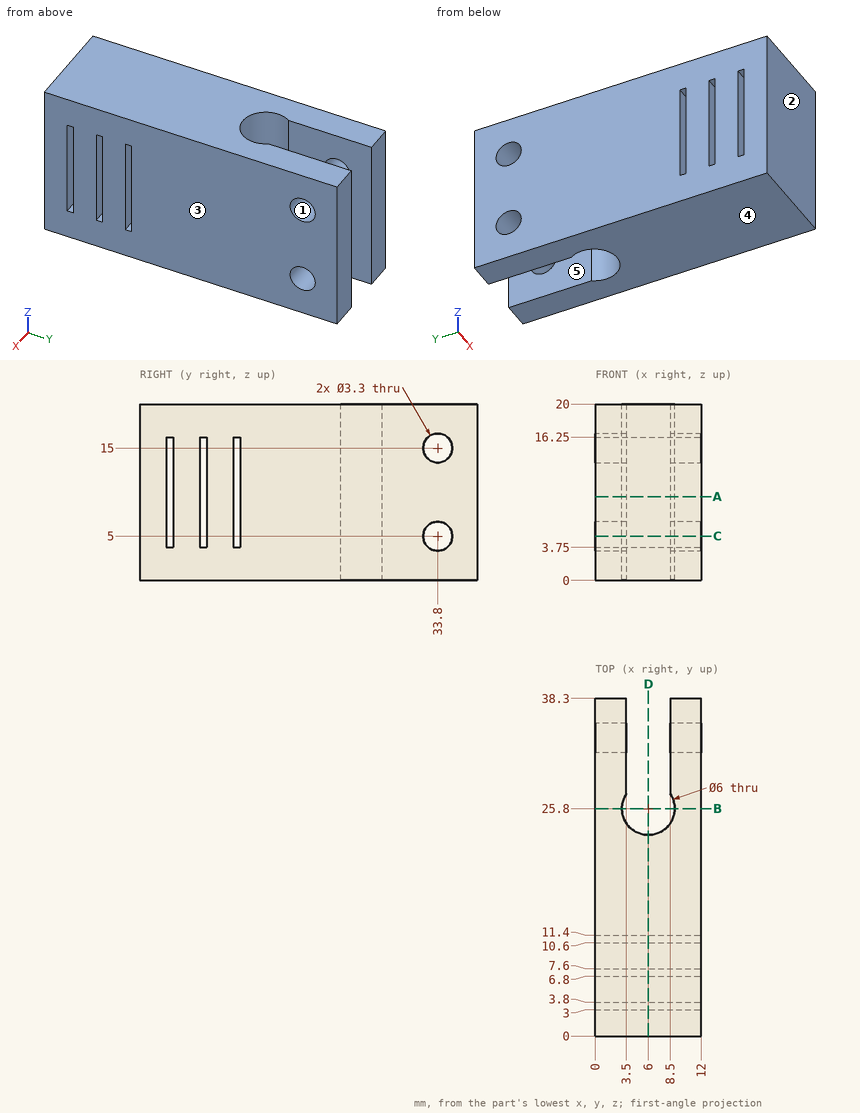
For this review, use the dimensioned drawing (mm, ordinates from the lowest corner) and the shaded views. A direction names the side the tool comes from. Give positions to 0.01 mm unless a question says otherwise; leave off trailing zeros. Order: outer loops, then holes, each group sorted by start corner. A loop starts at its lowest first (then second) coordinate and runs counter-clockwise, first axis right, second up.
1) Take a section at B-B (y = 25.8). Give the boundary of the cut face in (x, z), then the cut area to 3 significant figures.
2) Take a section at D-D (x = 6). Give the boundary of the cut face in (y, z).
3) Wall thickness on line 1 (Y direction, x = 6, z = 14.25); line 2 (Z direction, x = 10.8, y = 33.8); line 3 (Y direction, x = 2.7, z = 15): over which ranges is each line inside the solid? List them lowest first.
4) The part is to be moulded in two halves that separate along Y. For the marked faces 1, 2 and 3, say which applies: released by +Y, released by -Y, zero draft, split by the parting line, or undercut.
5) For the marked faces 4 and 5, list the 3-axis set-ups (+Z, -Z, +X, -X, +Y, -Y) from which the entire face can be reached by the end or side of a thin tool; tool diameter is ignored.
6) Take a section at A-A (z = 9.5). Give the boundary of the cut face in (x, y), then the cut area to 3 significant figures.
7) Take a section at C-C (z = 5). Give the boundary of the cut face in (x, y), then the cut area to 3 significant figures.
8) Insertion check: pin 1 (2 mm diameter, centred on x = 6, z = 13.5, fed in from +Y); pin 2 (3 mm diameter, centred on x = 5.5, z = 4, fed in from +Y). Each pin has a flat end and moves straight along its axis. Give the tip position at first contact, or say it passes through.
Derived:
1. outline: (0, 0) - (3, 0) - (3, 20) - (0, 20) - close; (9, 0) - (12, 0) - (12, 20) - (9, 20) - close
1. area: 120 mm2
2. outline: (0, 0) - (22.8, 0) - (22.8, 20) - (0, 20) - close; hole (3, 3.75) - (3.8, 3.75) - (3.8, 16.25) - (3, 16.25) - close; hole (6.8, 3.75) - (7.6, 3.75) - (7.6, 16.25) - (6.8, 16.25) - close; hole (10.6, 3.75) - (11.4, 3.75) - (11.4, 16.25) - (10.6, 16.25) - close
3. line 1: y = 0 to 3, 3.8 to 6.8, 7.6 to 10.6, 11.4 to 22.8
3. line 2: z = 0 to 3.35, 6.65 to 13.35, 16.65 to 20
3. line 3: y = 0 to 3, 3.8 to 6.8, 7.6 to 10.6, 11.4 to 32.15, 35.45 to 38.3
4. face 1: undercut
4. face 2: released by -Y
4. face 3: zero draft
5. face 4: -Z, +X, -X, +Y, -Y
5. face 5: +Z, -Z, +Y
6. outline: (0, 0) - (12, 0) - (12, 3) - (0, 3) - close; (0, 3.8) - (12, 3.8) - (12, 6.8) - (0, 6.8) - close; (0, 7.6) - (12, 7.6) - (12, 10.6) - (0, 10.6) - close; (0, 11.4) - (12, 11.4) - (12, 38.3) - (8.5, 38.3) - (8.5, 27.46) arc R3 cw (long way) to (3.5, 27.46) - (3.5, 38.3) - (0, 38.3) - close
6. area: 353 mm2
7. outline: (0, 0) - (12, 0) - (12, 3) - (0, 3) - close; (0, 3.8) - (12, 3.8) - (12, 6.8) - (0, 6.8) - close; (0, 7.6) - (12, 7.6) - (12, 10.6) - (0, 10.6) - close; (0, 11.4) - (12, 11.4) - (12, 32.15) - (8.5, 32.15) - (8.5, 27.46) arc R3 cw (long way) to (3.5, 27.46) - (3.5, 32.15) - (0, 32.15) - close; (0, 35.45) - (3.5, 35.45) - (3.5, 38.3) - (0, 38.3) - close; (8.5, 35.45) - (12, 35.45) - (12, 38.3) - (8.5, 38.3) - close
7. area: 330 mm2
8. pin 1: stops at y = 22.97
8. pin 2: stops at y = 23.56
